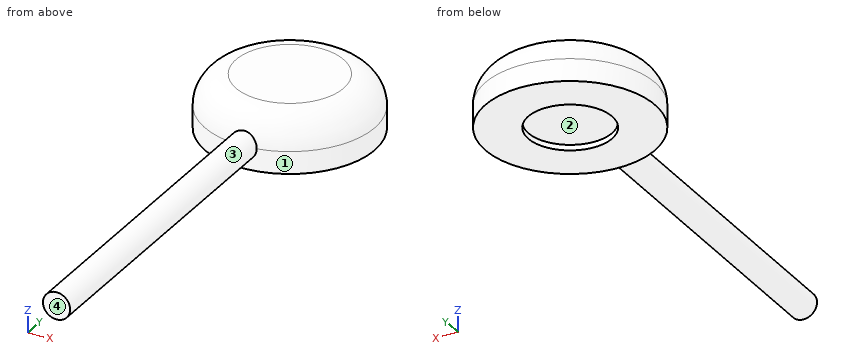
```python
from build123d import *

# Parameters (mm, degrees)
F0_R     = 11.735047
F1_DEPTH = 7.366
F2_R     = 4.292472
F3_R     = 5.7912
F4_DEPTH = 0.762
F5_R     = 1.875011
F6_DEPTH = 57.912


with BuildPart() as f1:
    # F0 (on Top) → F1 (new body)
    with BuildSketch(Plane.XY):
        Circle(F0_R)
    extrude(amount=F1_DEPTH)

    # F2
    f2_edges = [f1.edges().sort_by_distance(p)[0] for p in [
        (-11.735047, 0, 7.366),
    ]]
    fillet(f2_edges, radius=F2_R)

    # F3 (on face) → F4 (cut)
    with BuildSketch(Plane(origin=(0, 0, 0), x_dir=(1, 0, 0), z_dir=(0, 0, -1))):
        Circle(F3_R)
    extrude(amount=-F4_DEPTH, mode=Mode.SUBTRACT)

    # F5 (on Front) → F6 (join)
    with BuildSketch(Plane.XZ):
        with Locations((0, 3.073911)):
            Circle(F5_R)
    extrude(amount=F6_DEPTH)


solid = f1.part
```
For this review, take the finished solid that the model builds, in its own axes (mm). Face numbers are marked on the shaded views. Give positions to 0.01 mm unless a question says otherwise; leave off trailing zeros. Write each loop counter-clockwise with the first axis right and the second up, starting at its lowest first coordinate (ties: lowest second). Pieces come first, ordered by that corner, then holes. Notation, with made-up numbers: M 75.25,73 L 129.25,73 A25 cw 129.25,103 Z; hole C 83.5,62 d8. An arc over 180 degrees is marked long. Answer as a JSON object with one key per item and string values. Group by question number.
Item 1: Consider section D-D on z = 4. Write out the cut boundary in (x, y).
Item 2: For probe 1 along Y at (x, z) = (0, 0.6); probe 2 along X at (y, z) = (-31.5, 3.25), list the stretches that pass through material, from the lowest coordinate up. Write a range as [from, to].
Item 3: Consider section C-C on z = 6.75. Write out the cut boundary in (x, y), plus the area to 3 significant figures.
Item 4: Consider section A-A on x = 0. Write out the cut boundary in (y, z).
Item 5: Consider section B-B on y = 0. Write out the cut boundary in (x, z).
Item 6: Draft analysis for pull direction Y (two halves, no side actions). For the marked faces 1, 2, 3 and 4, state which applies: +Y half, -Y half, draft (parallel to the pull), parting line (faces both ways), or undercut.
Item 7: For pin 1 Ø4 at (y, z) = (-37.5, 6) entering from +X; pin 2 Ø6 at (x, y) = (0, -1) entering from -Z, all flat-tipped, find the tip position at first contact; note any pin that passes through.
Check result:
{
 "1": {"outline": "M -1.63,-57.91 L 1.63,-57.91 L 1.63,-11.52 A11.63 ccw long -1.63,-11.52 Z"},
 "2": {"probe 1": "y = [-11.74, -5.79], [5.79, 11.74]", "probe 2": "x = [-1.87, 1.87]"},
 "3": {"outline": "C 0,0 d19.32", "area": "293 mm^2"},
 "4": {"outline": "M -57.91,1.2 L -11.74,1.2 L -11.74,0 L -5.79,0 L -5.79,0.76 L 5.79,0.76 L 5.79,0 L 11.74,0 L 11.74,3.07 A4.29 ccw 7.44,7.37 L -7.44,7.37 A4.29 ccw -11.3,4.95 L -57.91,4.95 Z"},
 "5": {"outline": "M -11.74,0 L -5.79,0 L -5.79,0.76 L 5.79,0.76 L 5.79,0 L 11.74,0 L 11.74,3.07 A4.29 ccw 7.44,7.37 L -7.44,7.37 A4.29 ccw -11.74,3.07 Z"},
 "6": {"face 1": "parting line", "face 2": "undercut", "face 3": "draft", "face 4": "-Y half"},
 "7": {"pin 1": "stops at x = 1.63", "pin 2": "stops at z = 0.76"}
}
